```python
from build123d import *

# Parameters (mm, degrees)
BASE_4_R              = 1.5
BASE_4_R_2            = 0.75
BOSS_EXTRUDE5_DEPTH   = 3
BOSS_EXTRUDE5_2_DEPTH = 3
BASE_W                = 13.5
BASE_H                = 1
BOSS_EXTRUDE7_DEPTH   = 6.5
BASE_7_R              = 1.5
BASE_7_R_2            = 3
BOSS_EXTRUDE8_DEPTH   = 1
BOSS_EXTRUDE9_DEPTH   = 3
SLIT_W                = 10
SLIT_H                = 2
CUT_EXTRUDE2_DEPTH    = 6.5


with BuildPart() as part:
    # Base_4 → Boss-Extrude5 (new body)
    with BuildSketch(Plane(origin=(0, 0, 0), x_dir=(1, 0, 0), z_dir=(0, 1, 0))):
        with Locations(Location((-12, -12, 0), (0, 0, 270))):
            Circle(BASE_4_R)
        with Locations(Location((-12, -12, 0), (0, 0, 270))):
            Circle(BASE_4_R_2, mode=Mode.SUBTRACT)
    extrude(amount=BOSS_EXTRUDE5_DEPTH)



with BuildPart() as body_2:
    # Base_4 → Boss-Extrude5 2 (new body)
    with BuildSketch(Plane(origin=(0, 0, 0), x_dir=(1, 0, 0), z_dir=(0, 1, 0))):
        with Locations(Location((12, -12, 0), (0, 0, 270))):
            Circle(BASE_4_R)
        with Locations(Location((12, -12, 0), (0, 0, 270))):
            Circle(BASE_4_R_2, mode=Mode.SUBTRACT)
    extrude(amount=BOSS_EXTRUDE5_2_DEPTH)


with BuildPart() as body_3:
    # Base → Boss-Extrude7 (new body)
    with BuildSketch(Plane(origin=(0, 0, 0), x_dir=(1, 0, 0), z_dir=(0, 1, 0))):
        with Locations((0, 16)):
            Rectangle(BASE_W, BASE_H)
    extrude(amount=BOSS_EXTRUDE7_DEPTH)


with BuildPart() as part_1:
    add(part.part)

    add(body_2.part)  # Boss-Extrude8 merges body 2

    add(body_3.part)  # Boss-Extrude8 merges body 3
    # Base_7 → Boss-Extrude8 (add)
    with BuildSketch(Plane(origin=(0, 0, 0), x_dir=(1, 0, 0), z_dir=(0, 1, 0))):
        with BuildLine():
            ThreePointArc((14, 15), (13.560660172, 16.060660172), (12.5, 16.5))
            Line((12.5, 16.5), (6.75, 16.5))
            Line((6.75, 16.5), (6.75, 15.5))
            Line((6.75, 15.5), (-6.75, 15.5))
            Line((-6.75, 15.5), (-6.75, 16.5))
            Line((-6.75, 16.5), (-12.5, 16.5))
            ThreePointArc((-12.5, 16.5), (-13.560660172, 16.060660172), (-14, 15))
            Line((-14, 15), (-14, -15))
            ThreePointArc((-14, -15), (-13.560660172, -16.060660172), (-12.5, -16.5))
            Line((-12.5, -16.5), (12.5, -16.5))
            ThreePointArc((12.5, -16.5), (13.560660172, -16.060660172), (14, -15))
            Line((14, -15), (14, 15))
        make_face()
        with Locations(Location((-12, -12, 0), (0, 0, 270))):
            Circle(BASE_7_R, mode=Mode.SUBTRACT)
        with Locations(Location((0, -5, 0), (0, 0, 270))):
            Circle(BASE_7_R_2, mode=Mode.SUBTRACT)
        with Locations(Location((12, -12, 0), (0, 0, 270))):
            Circle(BASE_7_R, mode=Mode.SUBTRACT)
        with Locations(Location((0, 5, 0), (0, 0, 270))):
            Circle(BASE_7_R_2, mode=Mode.SUBTRACT)
    extrude(amount=BOSS_EXTRUDE8_DEPTH)

    # Base_8 → Boss-Extrude9 (add)
    with BuildSketch(Plane(origin=(0, 0, 0), x_dir=(1, 0, 0), z_dir=(0, 1, 0))):
        with BuildLine():
            Line((-5, -9.5), (5, -9.5))
            ThreePointArc((5, -9.5), (5.5, -10), (5, -10.5))
            Line((5, -10.5), (-5, -10.5))
            ThreePointArc((-5, -10.5), (-5.5, -10), (-5, -9.5))
        make_face()
        with BuildLine():
            Line((-5, 10.5), (5, 10.5))
            ThreePointArc((5, 10.5), (5.5, 10), (5, 9.5))
            Line((5, 9.5), (-5, 9.5))
            ThreePointArc((-5, 9.5), (-5.5, 10), (-5, 10.5))
        make_face()
    extrude(amount=BOSS_EXTRUDE9_DEPTH)

    # slit → Cut-Extrude2 (cut)
    with BuildSketch(Plane.XY.offset(-15.5)):
        with Locations((0, 4)):
            Rectangle(SLIT_W, SLIT_H)
    extrude(amount=-CUT_EXTRUDE2_DEPTH, mode=Mode.SUBTRACT)


solid = part_1.part
```
Geometry check sheet. Reference: the model listing, model coordinates, mm. A direction names the side the tool comes from. Coordinates: 2 decimals unless noted, no trailing zeros. Write each loop counter-clockwise with the first axis right and the second up, starting at its lowest first coordinate (ties: lowest second). Pieces come first, ordered by that corner, then holes. Notation, with made-up numbers: M 6.25,57.25 L 61.25,57.25 A22 ccw 61.25,94.25 Z; hole C 33,5.25 d3. An arc over 180 degrees is marked long. One line per item, written item: value. Start each with the question number.
(1) Release check for a two-part mould opening along Y. For faces 4 (the face through (-12, 3, 11)), 5 (the face through (-5, 4, -16)), 6 (the face through (-0.2, 0.5, 16.5)) record: released by +Y, released by -Y, zero draft, split by the parting line, or undercut.
(2) Scan lines: line 1 along X through (y, z) = (1.1, 12); line 2 along Z through (x, y) = (-2.75, 0.75); line 3 along X through (y, z) = (0.4, -5). Record each from-to range of solid material in increasing order. Write a range as [from, to].
(3) Sectioned sample at D-D, the plane z = -5. Enter the section's corners in (x, y).
(4) Depth check by flat-ended pin: pin 1 (1.6 mm diameter, centred on x = 1, y = 4.5, fed in from +Z); pin 2 (1.1 mm diameter, centred on y = 4, z = -16, fed in from -X); pin 3 (14 mm diameter, centred on x = -4.5, z = 7, fed in from +Y). Enter the tip coordinate at first touch or a pass-through.
(5) Sectioned sample at C-C, the plane y = 2. Enter the section's corners in (x, z), and give its area (3 significant figures).
(6) Sectioned sample at B-B, the plane x = -12. Enter the section's corners in (y, z).
(7) Sectioned sample at A-A, the plane z = 12. Enter the section's corners in (x, y), and give its area (3 significant figures).
(8) Tool access check on faces 1 (the face through (5.5, 2, -10)), 2 (the face through (0, 2, 10.5)), 3 (the face through (-11.93, 1.99, 10.5)). Record the directions out of +Z, -Z, +X, -X, +Y, -Y that give a thin tool (end or side, any length) a straight path to the whole face; none if there is none.
Filled sheet:
1. face 4: released by +Y
1. face 5: undercut
1. face 6: zero draft
2. line 1: [-13.5, -12.75], [-11.25, -10.5], [10.5, 11.25], [12.75, 13.5]
2. line 2: [-16.5, -6.2], [-3.8, 3.8], [6.2, 16.5]
2. line 3: [-14, -3], [3, 14]
3. outline: M -14,0 L -3,0 L -3,1 L -14,1 Z; M 3,0 L 14,0 L 14,1 L 3,1 Z
4. pin 1: z = -15.5
4. pin 2: x = -6.75
4. pin 3: y = 3
5. outline: C -12,12 d3; M -6.75,-16.5 L 6.75,-16.5 L 6.75,-15.5 L -6.75,-15.5 Z; M -5,-10.5 L 5,-10.5 A0.5 ccw 5,-9.5 L -5,-9.5 A0.5 ccw Z; M -5,9.5 L 5,9.5 A0.5 ccw 5,10.5 L -5,10.5 A0.5 ccw Z; C 12,12 d3; hole C -12,12 d1.5; hole C 12,12 d1.5
5. area: 45.7 mm²
6. outline: M 0,-16.5 L 1,-16.5 L 1,10.5 L 3,10.5 L 3,11.25 L 0,11.25 Z; M 0,12.75 L 3,12.75 L 3,13.5 L 1,13.5 L 1,16.5 L 0,16.5 Z
7. outline: M -14,0 L -12.75,0 L -12.75,3 L -13.5,3 L -13.5,1 L -14,1 Z; M -11.25,0 L 11.25,0 L 11.25,3 L 10.5,3 L 10.5,1 L -10.5,1 L -10.5,3 L -11.25,3 Z; M 12.75,0 L 14,0 L 14,1 L 13.5,1 L 13.5,3 L 12.75,3 Z
7. area: 31.0 mm²
8. face 1: +X, +Y
8. face 2: +Z, +Y
8. face 3: +Y
